from build123d import *

# Parameters (mm, degrees)
SKETCH1_W           = 230
SKETCH1_H           = 129
BOSS_EXTRUDE1_DEPTH = 2
SKETCH2_W           = 37
SKETCH2_H           = 22
SKETCH2_W_2         = 57
SKETCH2_H_2         = 36
SKETCH2_W_3         = 30
SKETCH2_H_3         = 80
CUT_EXTRUDE1_DEPTH  = 3
SKETCH3_R           = 1.65
SKETCH3_R_2         = 1.6
CUT_EXTRUDE2_DEPTH  = 10
FILLET1_R           = 4


with BuildPart() as part:
    # Sketch1 → Boss-Extrude1 (new body)
    with BuildSketch(Plane(origin=(0, 0, 0), x_dir=(1, 0, 0), z_dir=(0, 1, 0))):
        with Locations((115, 64.5)):
            Rectangle(SKETCH1_W, SKETCH1_H)
    extrude(amount=BOSS_EXTRUDE1_DEPTH)

    # Sketch2 → Cut-Extrude1 (cut, through all)
    with BuildSketch(Plane(origin=(0, 2, 0), x_dir=(1, 0, 0), z_dir=(0, 1, 0))):
        with Locations((18.5, 118)):
            Rectangle(SKETCH2_W, SKETCH2_H)
        with Locations((28.5, 18)):
            Rectangle(SKETCH2_W_2, SKETCH2_H_2)
        with Locations((211.5, 118)):
            Rectangle(SKETCH2_W, SKETCH2_H)
        with Locations((201.5, 18)):
            Rectangle(SKETCH2_W_2, SKETCH2_H_2)
        with Locations((115, 40)):
            Rectangle(SKETCH2_W_3, SKETCH2_H_3)
    extrude(amount=-CUT_EXTRUDE1_DEPTH, mode=Mode.SUBTRACT)

    # Sketch3 → Cut-Extrude2 (cut)
    with BuildSketch(Plane.XZ):
        with Locations((5, -41)):
            Circle(SKETCH3_R)
        with Locations((5, -102)):
            Circle(SKETCH3_R)
        with Locations((95, -5)):
            Circle(SKETCH3_R)
        with Locations((95, -93)):
            Circle(SKETCH3_R)
        with Locations((95, -123)):
            Circle(SKETCH3_R)
        with Locations((135, -93)):
            Circle(SKETCH3_R)
        with Locations((135, -5)):
            Circle(SKETCH3_R)
        with Locations((135, -123)):
            Circle(SKETCH3_R)
        with Locations((225, -41)):
            Circle(SKETCH3_R)
        with Locations((225, -102)):
            Circle(SKETCH3_R)
        with Locations((61, -34)):
            Circle(SKETCH3_R)
        with Locations((61, -4)):
            Circle(SKETCH3_R)
        with Locations((169, -34)):
            Circle(SKETCH3_R)
        with Locations((169, -4)):
            Circle(SKETCH3_R)
        with Locations((45, -125)):
            Circle(SKETCH3_R_2)
        with Locations((185, -125)):
            Circle(SKETCH3_R_2)
    extrude(amount=-CUT_EXTRUDE2_DEPTH, mode=Mode.SUBTRACT)

    # Fillet1
    fillet1_edges = [part.edges().sort_by_distance(p)[0] for p in [
        (0, 1, -36),
        (57, 1, -36),
        (57, 1, 0),
        (230, 1, -107),
        (193, 1, -129),
        (230, 1, -36),
        (173, 1, 0),
        (173, 1, -36),
        (100, 1, 0),
        (100, 1, -80),
        (130, 1, -80),
        (130, 1, 0),
        (0, 1, -107),
        (37, 1, -129),
    ]]
    fillet(fillet1_edges, radius=FILLET1_R)


solid = part.part
For this review, take the finished solid that the model builds, in its own axes (mm). A direction names the side the tool comes from. Round coordinates to 2 decimals unless told otherwise and drop trailing zeros. Loops run counter-clockwise (first coordinate to the right, second up) from the corner with the lowest first, then second, coordinate; pieces in that order, holes last. Notation, with made-up numbers: (57, 30.25) - (64, 30.25) arc R19 ccw to (64, 37.25) - close; hole circle Ø2 at (29.25, -36). An arc over 180 degrees is marked (long way). One line per item, written item: value. Start each with the question number.
Item 1: Take a section at D-D (x = 34). Give the boundary of the cut face in (y, z).
Item 2: Clearance check with flat-ended pins moving along their axes: pin 1 Ø0.6 at (y, z) = (0.5, -13) entering from -X; pin 2 Ø0.6 at (y, z) = (1, -37) entering from -X. State where each tip first meets the part, or that it passes through.
Item 3: Take a section at C-C (y = 0.45). State how many separate pieces and enclosed holes the cut face has, plus the area to 3 significant figures.
Item 4: Take a section at B-B (z = -29.5). Give the boundary of the cut face in (x, y).
Item 5: For faces 4 (the cylindrical face through (55.797, 0.986, -34.859)), 5 (the cylindrical face through (128.797, 0.986, -78.859)), list the 3-axis set-ups (+Z, -Z, +X, -X, +Y, -Y) from which the entire face can be reached by the end or side of a thin tool; tool diameter is ignored.
Item 6: The part is to be moulded in two halves that separate along X. For faces 1 (the cylindrical face through (131.141, 0.986, -1.203)), 2 (the cylindrical face through (58.141, 0.986, -1.203)), 3 (the flat face through (139, 2, -65)), say which applies: +X half, -X half, draft (parallel to the pull), parting line (faces both ways), or undercut.
Item 7: Take a section at A-A (z = -58). Give the boundary of the cut face in (x, y).
Item 8: For L1, parallel to Z at x = 5, y = 1.5; L2, parallel to Z at x = 61, y = 0.6; L3, parallel to Z at x = 135, y = 0.65, list the stretches that pass through material, from the lowest coordinate up.
Answer below:
1. outline: (0, -107) - (2, -107) - (2, -36) - (0, -36) - close
2. pin 1: stops at x = 57
2. pin 2: stops at x = 1.05
3. separate pieces: 1
3. enclosed holes: 16
3. area: 21,400 mm2
4. outline: (57, 0) - (100, 0) - (100, 2) - (57, 2) - close; (130, 0) - (173, 0) - (173, 2) - (130, 2) - close
5. face 4: +Z, -X, +Y, -Y
5. face 5: +Z, +Y, -Y
6. face 1: undercut
6. face 2: -X half
6. face 3: draft
7. outline: (0, 0) - (100, 0) - (100, 2) - (0, 2) - close; (130, 0) - (230, 0) - (230, 2) - (130, 2) - close
8. L1: z = -107 to -103.65, -100.35 to -42.65, -39.35 to -36
8. L2: z = -129 to -35.65, -32.35 to -5.65, -2.35 to 0
8. L3: z = -129 to -124.65, -121.35 to -94.65, -91.35 to -6.65, -3.35 to 0
